Could you check a few things on this drawing? It's one solid part, dimensions in mm from its lowest x, y, z. A direction names the side the tool comes from. Give positions to 0.01 mm unless a question says otherwise; leave off trailing zeros. Write each loop counter-clockwise with the first axis right and the second up, starting at its lowest first coordinate (ties: lowest second). Pieces come first, ordered by that corner, then holes. Notation, with made-up numbers: M 72,-18.75 L 93,-18.75 A34 ccw 93,16.25 Z; hole C 76,72.5 d2. An arc over 180 degrees is marked long. Use CSV: the item, a comma, the result in double quotes. Start each with the question number.
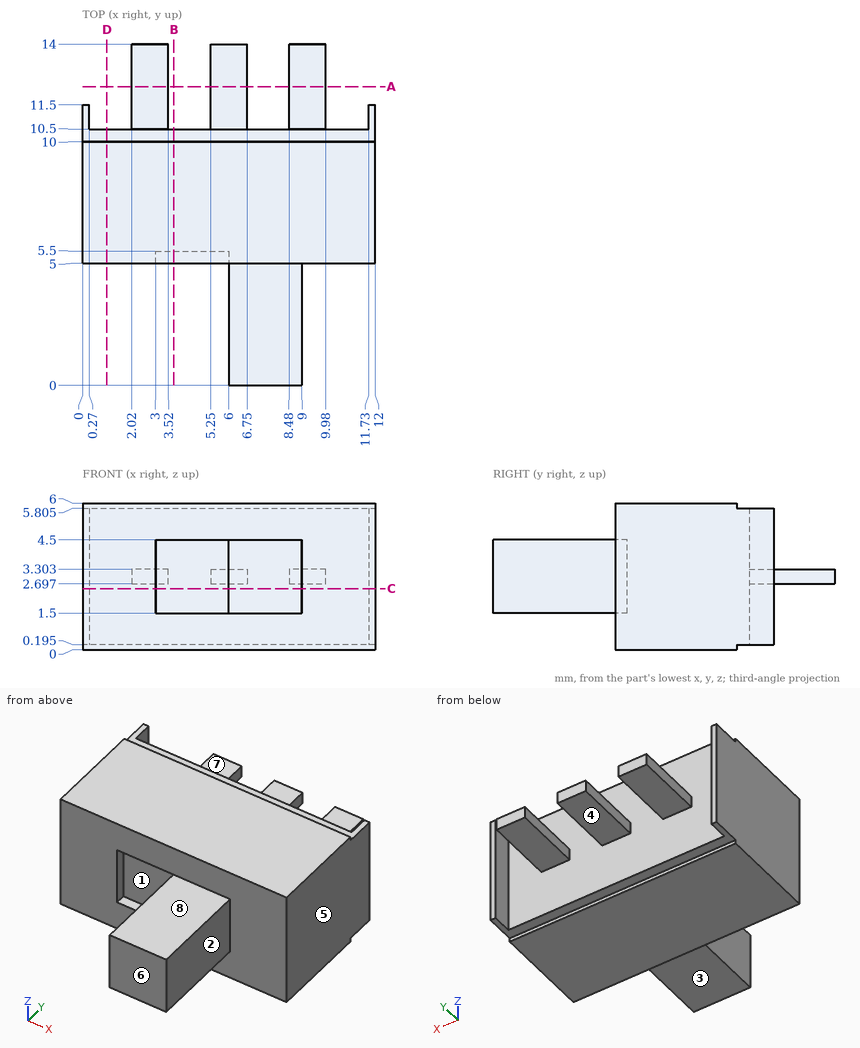
(1) I want a section at B-B (x = 3.75). Write out the boundary of the cut face in (y, z) (3 decimals), and give its area (3 significant figures).
(2) I want a section at C-C (z = 2.5). Write out the boundary of the cut face in (x, y).
(3) I want a section at D-D (x = 1). Write out the boundary of the cut face in (y, z) (3 decimals), and give its area (3 significant figures).
(4) Please list where these lines run through material, in increasing order: L1, parallel to Y at x = 5.5, z = 0.65; L2, parallel to Y at x = 4.75, z = 3.25; L3, parallel to Z at x = 9, y = 12.75. Write a range as [from, to].
(5) Thinking about a two-plate mould opening in Z: for the marked faces 1, 2 and 3, which applies, released by +Z, released by -Z, zero draft, split by the parting line, or undercut?
(6) Which directions (+Z, -Z, +X, -X, +Y, -Y) give clear straight access to the entire face, cutting with the end or side of a thin tool? Please do the marked faces 4, 5, 6, 7 and 8.
(7) Will these pins go through, and if not, where does the flat tip stop? pin 1 Ø1.2 at (x, y) = (4, 11) entering from -Z (3 decimals); pin 2 Ø2.5 at (y, z) = (2, 3) entering from +X; pin 3 Ø0.7 at (y, z) = (12, 3) entering from -X; pin 4 Ø3 at (x, y) = (5.5, 5) entering from -Z.
(8) I want a section at A-A (y = 12.25). Write out the boundary of the cut face in (x, z).
Geometry results:
1,outline,"M 5,0 L 10,0 L 10,0.195 L 10.5,0.195 L 10.5,5.805 L 10,5.805 L 10,6 L 5,6 L 5,4.5 L 5.5,4.5 L 5.5,1.5 L 5,1.5 Z"
1,area,"31.3 mm2"
2,outline,"M 0,5 L 3,5 L 3,5.5 L 6,5.5 L 6,0 L 9,0 L 9,5 L 12,5 L 12,11.5 L 11.73,11.5 L 11.73,10.5 L 0.27,10.5 L 0.27,11.5 L 0,11.5 Z"
3,outline,"M 5,0 L 10,0 L 10,0.195 L 10.5,0.195 L 10.5,5.805 L 10,5.805 L 10,6 L 5,6 Z"
3,area,"32.8 mm2"
4,L1,"y = [5, 10.5]"
4,L2,"y = [5.5, 10.5]"
4,L3,"z = [2.7, 3.3]"
5,face 1,"undercut"
5,face 2,"zero draft"
5,face 3,"released by -Z"
6,face 4,"-Z, +Y"
6,face 5,"+Z, -Z, +X, +Y, -Y"
6,face 6,"+Z, -Z, +X, -X, -Y"
6,face 7,"+Z, +Y"
6,face 8,"+Z, +X, -X, -Y"
7,pin 1,"stops at z = 0.195"
7,pin 2,"stops at x = 9"
7,pin 3,"stops at x = 2.02"
7,pin 4,"stops at z = 0"
8,outline,"M 2.02,2.7 L 3.52,2.7 L 3.52,3.3 L 2.02,3.3 Z; M 5.25,2.7 L 6.75,2.7 L 6.75,3.3 L 5.25,3.3 Z; M 8.48,2.7 L 9.98,2.7 L 9.98,3.3 L 8.48,3.3 Z"
